Build history of the part. All positions in model axes, mm. A direction names the side the tool comes from. Give positions to 0.01 mm unless a question says otherwise; leave off trailing zeros. Write each loop counter-clockwise with the first axis right and the second up, starting at its lowest first coordinate (ties: lowest second). Pieces come first, ordered by that corner, then holes. Notation, with made-up numbers: M -9.5,48 L -2.5,48 A24 ccw -2.5,71 Z; hole C 59.5,-16.5 d6. An arc over 180 degrees is marked long. Return JSON: item names as keys, results as strings. Group by question number.
Q1. Pull direction X, two halves, no side cores. Call faces 1 (the cylindrical face through (-9, 5.86, 1.97)), 2 (the flat face through (-17, 0, 0)), 3 (the flat face through (-1.2, -9, 3)), 4 (the flat face through (-8.1, 11, 3)): +X half, -X half, draft (parallel to the pull), parting line (faces both ways), or undercut.
Q2. Wall check: probe 1 along Y at (x, z) = (-5.75, 5.6); probe 2 along X at (y, z) = (9.25, 2.5); probe 3 along Z at (x, y) = (-9.5, -5). Give the ranges that are in metal, low to high.
Q3. Band-saw the part on C-C, the plane z = 5.6. Count the separate pieces of the cut face and the enclosed holes in it, then the cut area to 3 significant figures.
Q4. Band-saw the part on A-A, the plane y = 12. Give the cut face in (x, z).
Q5. Band-saw the part on D-D, the plane y = -12. Give the cut face in (x, z).
Q6. Flat gauge pins, fed straight in: pin 1 Ø3 at (y, z) = (-11.5, 6) entering from -X; pin 2 Ø5.5 at (x, y) = (-25, 2.5) entering from +Z; pin 3 Ø0.8 at (x, y) = (-29.5, 14.5) entering from +Z. Where does each tip first touch, or does it go through?
Q7. Band-saw the part on B-B, the plane x = -27. Give the cut face in (y, z), then the cut area to 3 significant figures.
Q8. Tool access for faces 5 (the cylindrical face through (-33.123, 14.704, 2.028)), 6 (the cylindrical face through (-24.54, 5.9, 1.97)), 7 (the flat face through (-32.393, -13, 4)), 8 (the flat face through (-17, -5, 2)): list every direction of +Z, -Z, +X, -X, +Y, -Y with a clear straight run to the whole face (end or side of a thin tool).
from build123d import *

# Parameters (mm, degrees)
BOSS_EXTRUDE1_DEPTH             = 4
FILLET1_R                       = 1
BOSS_EXTRUDE3_REACH             = 25.017
SKETCH5_R                       = 3
SKETCH5_R_2                     = 1.6
BOSS_EXTRUDE3_DIRECTION_2_REACH = 25.017
CUT_EXTRUDE2_START              = -8.6000001
CUT_EXTRUDE2_DEPTH              = 6.0000001


# Read off the part's stored shape, not the designer's step: Cut-Extrude2
with BuildPart() as part:
    # Sketch1 → Boss-Extrude1 (new body)
    with BuildSketch(Plane.XY):
        with BuildLine():
            Line((-25.399999997, 14.999666663), (-25.399999997, 7.999666663))
            ThreePointArc((-25.399999997, 7.999666663), (-24.52132034, 5.878346319), (-22.399999997, 4.999666663))
            Line((-22.399999997, 4.999666663), (-11.099999997, 4.999666663))
            ThreePointArc((-11.099999997, 4.999666663), (-8.978679653, 5.878346319), (-8.099999997, 7.999666663))
            Line((-8.099999997, 7.999666663), (-8.099999997, 14.999666663))
            Line((-8.099999997, 14.999666663), (-0.099999997, 14.999666663))
            Line((-0.099999997, 14.999666663), (0, 0))
            Line((0, 0), (-0.2, 0))
            ThreePointArc((-0.2, 0), (-0.907106781, -0.292893219), (-1.2, -1))
            Line((-1.2, -1), (-1.2, -14.999666663))
            Line((-1.2, -14.999666663), (-7.900000003, -14.999666663))
            Line((-7.900000003, -14.999666663), (-7.900000003, -7.999666663))
            ThreePointArc((-7.900000003, -7.999666663), (-8.77867966, -5.878346319), (-10.900000003, -4.999666663))
            Line((-10.900000003, -4.999666663), (-22.500000003, -4.999666663))
            ThreePointArc((-22.500000003, -4.999666663), (-24.621320347, -5.878346319), (-25.500000003, -7.999666663))
            Line((-25.500000003, -7.999666663), (-25.500000003, -14.999666663))
            Line((-25.500000003, -14.999666663), (-32.300000003, -14.999666663))
            Line((-32.300000003, -14.999666663), (-32.39337598, -0.993276115))
            ThreePointArc((-32.39337598, -0.993276115), (-32.688706434, -0.290384923), (-33.39363154, 5.7325e-05))
            Line((-33.39363154, 5.7325e-05), (-33.6, 0))
            Line((-33.6, 0), (-33.399999997, 14.999666663))
            Line((-33.399999997, 14.999666663), (-25.399999997, 14.999666663))
        make_face()
    extrude(amount=BOSS_EXTRUDE1_DEPTH)

    # Fillet1
    fillet1_edges = [part.edges().sort_by_distance(p)[0] for p in [
        (-7.900000003, -14.999666663, 2),
        (-25.500000003, -14.999666663, 2),
        (-0.099999997, 14.999666663, 2),
        (-8.099999997, 14.999666663, 2),
        (-25.399999997, 14.999666663, 2),
        (-33.399999997, 14.999666663, 2),
        (-32.300000003, -14.999666663, 2),
        (-33.6, 0, 2),
        (-1.2, -14.999666663, 2),
        (0, 0, 2),
    ]]
    fillet(fillet1_edges, radius=FILLET1_R)

    # Boss-Extrude3: up to this plane
    boss_extrude3_end = Plane(origin=(-33.399999997, 14.999666663, 4), z_dir=(0.9999111190085467, -0.013332444752411323, 0))
    # Sketch5 → Boss-Extrude3 (add, up to the surface)
    with BuildSketch(Plane.ZY.offset(16.999999997), mode=Mode.PRIVATE) as boss_extrude3_sk1:
        with Locations(Location((5.6, 11.499666663, 0), (0, 0, 123.557309762))):
            Circle(SKETCH5_R)
        with Locations(Location((5.6, 11.499666663, 0), (0, 0, 90))):
            Circle(SKETCH5_R_2, mode=Mode.SUBTRACT)
    boss_extrude3_tool1 = split(extrude(boss_extrude3_sk1.sketch, amount=BOSS_EXTRUDE3_REACH, mode=Mode.PRIVATE), bisect_by=boss_extrude3_end, keep=Keep.BOTH, mode=Mode.PRIVATE)
    add(boss_extrude3_tool1.solids().sort_by_distance((-17, 9.070377, 7.211408))[0])
    # Sketch5 → Boss-Extrude3 (add, up to the surface)
    with BuildSketch(Plane.ZY.offset(16.999999997), mode=Mode.PRIVATE) as boss_extrude3_sk2:
        with Locations(Location((5.6, -11.499666663, 0), (0, 0, 90))):
            Circle(SKETCH5_R)
        with Locations(Location((5.6, -11.499666663, 0), (0, 0, 90))):
            Circle(SKETCH5_R_2, mode=Mode.SUBTRACT)
    boss_extrude3_tool2 = split(extrude(boss_extrude3_sk2.sketch, amount=BOSS_EXTRUDE3_REACH, mode=Mode.PRIVATE), bisect_by=boss_extrude3_end, keep=Keep.BOTH, mode=Mode.PRIVATE)
    add(boss_extrude3_tool2.solids().sort_by_distance((-17, -14.414814, 5.6))[0])

    # Boss-Extrude3 direction 2: up to this plane
    boss_extrude3_direction_2_end = Plane(origin=(-0.099999997, 14.999666663, 4), z_dir=(-0.9999777775323199, -0.006666666447507326, 0))
    # Sketch5 → Boss-Extrude3 direction 2 (add, up to the surface)
    with BuildSketch(Plane.ZY.offset(16.999999997), mode=Mode.PRIVATE) as boss_extrude3_direction_2_sk1:
        with Locations(Location((5.6, 11.499666663, 0), (0, 0, 123.557309762))):
            Circle(SKETCH5_R)
        with Locations(Location((5.6, 11.499666663, 0), (0, 0, 90))):
            Circle(SKETCH5_R_2, mode=Mode.SUBTRACT)
    boss_extrude3_direction_2_tool1 = split(extrude(boss_extrude3_direction_2_sk1.sketch, amount=-BOSS_EXTRUDE3_DIRECTION_2_REACH, mode=Mode.PRIVATE), bisect_by=boss_extrude3_direction_2_end, keep=Keep.BOTH, mode=Mode.PRIVATE)
    add(boss_extrude3_direction_2_tool1.solids().sort_by_distance((-17, 9.070377, 7.211408))[0])
    # Sketch5 → Boss-Extrude3 direction 2 (add, up to the surface)
    with BuildSketch(Plane.ZY.offset(16.999999997), mode=Mode.PRIVATE) as boss_extrude3_direction_2_sk2:
        with Locations(Location((5.6, -11.499666663, 0), (0, 0, 90))):
            Circle(SKETCH5_R)
        with Locations(Location((5.6, -11.499666663, 0), (0, 0, 90))):
            Circle(SKETCH5_R_2, mode=Mode.SUBTRACT)
    boss_extrude3_direction_2_tool2 = split(extrude(boss_extrude3_direction_2_sk2.sketch, amount=-BOSS_EXTRUDE3_DIRECTION_2_REACH, mode=Mode.PRIVATE), bisect_by=boss_extrude3_direction_2_end, keep=Keep.BOTH, mode=Mode.PRIVATE)
    add(boss_extrude3_direction_2_tool2.solids().sort_by_distance((-17, -14.414814, 5.6))[0])

    # Cut-Extrude2 outline → Cut-Extrude2 (cut)
    with BuildSketch(Plane(origin=(0, 0, 0), x_dir=(-1, 0, 0), z_dir=(0, 0, -1)).offset(CUT_EXTRUDE2_START)):
        Polygon((37.39337598, -0.993276115), (32.39337598, -0.993276115), (32.39337598, -8.499666663), (32.39337598, -14.499666663), (32.39337598, -14.999666663), (37.39337598, -14.999666663), align=None)
        with BuildLine():
            Line((26.399999997, 14.999666663), (7.099999997, 14.999666663))
            ThreePointArc((7.099999997, 14.999666663), (7.807106778, 14.706773444), (8.099999997, 13.999666663))
            Line((8.099999997, 13.999666663), (8.099999997, 7.999666663))
            ThreePointArc((8.099999997, 7.999666663), (8.978679653, 5.878346319), (11.099999997, 4.999666663))
            Line((11.099999997, 4.999666663), (22.399999997, 4.999666663))
            ThreePointArc((22.399999997, 4.999666663), (24.52132034, 5.878346319), (25.399999997, 7.999666663))
            Line((25.399999997, 7.999666663), (25.399999997, 13.999666663))
            ThreePointArc((25.399999997, 13.999666663), (25.692893216, 14.706773444), (26.399999997, 14.999666663))
        make_face()
        with BuildLine():
            Line((1.2, -13.999666663), (1.2, -1))
            Line((1.2, -1), (-2.8, -1))
            Line((-2.8, -1), (-2.8, -14.999666663))
            Line((-2.8, -14.999666663), (2.2, -14.999666663))
            ThreePointArc((2.2, -14.999666663), (1.492893219, -14.706773444), (1.2, -13.999666663))
        make_face()
        with BuildLine():
            ThreePointArc((7.900000003, -13.999666663), (7.607106784, -14.706773444), (6.900000003, -14.999666663))
            Line((6.900000003, -14.999666663), (26.500000003, -14.999666663))
            ThreePointArc((26.500000003, -14.999666663), (25.792893222, -14.706773444), (25.500000003, -13.999666663))
            Line((25.500000003, -13.999666663), (25.500000003, -7.999666663))
            ThreePointArc((25.500000003, -7.999666663), (24.621320347, -5.878346319), (22.500000003, -4.999666663))
            Line((22.500000003, -4.999666663), (10.900000003, -4.999666663))
            ThreePointArc((10.900000003, -4.999666663), (8.77867966, -5.878346319), (7.900000003, -7.999666663))
            Line((7.900000003, -7.999666663), (7.900000003, -13.999666663))
        make_face()
    extrude(amount=CUT_EXTRUDE2_DEPTH, mode=Mode.SUBTRACT)


solid = part.part
From the geometry:
{
 "1": {"face 1": "undercut", "face 2": "draft", "face 3": "+X half", "face 4": "undercut"},
 "2": {"probe 1": "y = -14.5 to -13.1, -9.9 to -8.5, 8.5 to 9.9, 13.1 to 14.5", "probe 2": "x = -33.48 to -25.4, -8.1 to -0.06", "probe 3": "z = 0 to 4"},
 "3": {"separate pieces": "8", "enclosed holes": "0", "area": "82.9 mm^2"},
 "4": {"outline": "M -33.44,0 L -25.4,0 L -25.4,4.08 L -33.44,4.08 Z; M -33.44,7.12 L -25.4,7.12 L -25.4,8.56 L -33.44,8.56 Z; M -8.1,0 L -0.08,0 L -0.08,4.08 L -8.1,4.08 Z; M -8.1,7.12 L -0.08,7.12 L -0.08,8.56 L -8.1,8.56 Z"},
 "5": {"outline": "M -32.39,2.64 L -32.32,2.64 L -32.32,0 L -25.5,0 L -25.5,4.08 L -32.39,4.08 Z; M -32.39,7.12 L -25.5,7.12 L -25.5,8.56 L -32.39,8.56 Z; M -7.9,0 L -1.2,0 L -1.2,4.08 L -7.9,4.08 Z; M -7.9,7.12 L -1.2,7.12 L -1.2,8.56 L -7.9,8.56 Z"},
 "6": {"pin 1": "stops at x = -32.39", "pin 2": "stops at z = 4", "pin 3": "stops at z = 7.1"},
 "7": {"outline": "M -15,0 L 15,0 L 15,4 L 14.04,4 A3 ccw long 8.96,4 L -8.96,4 A3 ccw long -14.04,4 L -15,4 Z; hole C -11.5,5.6 d3.2; hole C 11.5,5.6 d3.2", "area": "150 mm^2"},
 "8": {"face 5": "-Z, -X, +Y", "face 6": "+Z, -Z, +Y", "face 7": "+Z, -Z, -X, -Y", "face 8": "+Z, -Z, -Y"}
}
